```python
from build123d import *

# Parameters (mm, degrees)
SKETCH_1_W             = 372.5
SKETCH_1_H             = 50
SM_BASE_FLANGE_1_DEPTH = 8
OTHER_START            = -25
OTHER_1_DEPTH          = 50
OTHER_1_2_DEPTH        = 50
CHAMFER_1_SIZE         = 10
CUT_EXTRUDE_1_DEPTH    = 374.873307418
M8X1_251_D             = 6.8
M8X1_251_CSINK_D       = 8.5
M8X1_251_CSINK_ANGLE   = 90


# Read off the part's stored shape, not the designer's step: Изгиб1
# Sheet-metal steps are written as plain solids
with BuildPart() as part:
    # Sketch 1 → Базовая кромка1 (new body)
    with BuildSketch(Plane(origin=(0, 0, 0), x_dir=(1, 0, 0), z_dir=(0, 1, 0))):
        with Locations((-186.25, 0)):
            Rectangle(SKETCH_1_W, SKETCH_1_H)
    extrude(amount=SM_BASE_FLANGE_1_DEPTH)

    # Other 1 outline → Other 1 (cut)
    with BuildSketch(Plane.XY.offset(OTHER_START)):
        with BuildLine():
            Line((-306.372583002, 8), (-309.68629166, 4.68629166))
            ThreePointArc((-309.68629166, 4.68629166), (-314.877065168, 1.217927687), (-321, 2.25e-07))
            Line((-321, 2.25e-07), (0, 0))
            Line((0, 0), (0, 8))
            Line((0, 8), (-306.372583002, 8))
        make_face()
    extrude(amount=OTHER_1_DEPTH, mode=Mode.SUBTRACT)

    # Other 1 2 outline → Other 1 2 (add)
    with BuildSketch(Plane.XY.offset(OTHER_START)):
        with BuildLine():
            Line((-321, 8.000000225), (-306.372583002, 8))
            Line((-306.372583002, 8), (-296.715728655, 17.656854152))
            ThreePointArc((-296.715728655, 17.656854152), (-294.120341909, 19.391036132), (-291.058874503, 19.999999862))
            Line((-291.058874503, 19.999999862), (0, 20))
            Line((0, 20), (0, 28))
            Line((0, 28), (-291.058874503, 27.999999862))
            ThreePointArc((-291.058874503, 27.999999862), (-297.181809368, 26.782072393), (-302.372582904, 23.313708401))
            Line((-302.372582904, 23.313708401), (-315.343145909, 10.343145909))
            ThreePointArc((-315.343145909, 10.343145909), (-317.938532627, 8.608963948), (-321, 8.000000225))
        make_face()
    extrude(amount=OTHER_1_2_DEPTH)

    # Фаска1
    chamfer_1_edges = [part.edges().sort_by_distance(p)[0] for p in [
        (-372.5, 4, -25),
        (-372.5, 4, 25),
    ]]
    chamfer(chamfer_1_edges, length=CHAMFER_1_SIZE)

    # Эскиз4 → Вытянуть1 (cut, through all)
    with BuildSketch(Plane(origin=(0, 8, 0), x_dir=(1, 0, 0), z_dir=(0, 1, 0))):
        with BuildLine():
            Line((-348.5, 8.5), (-372.5, 8.5))
            Line((-372.5, 8.5), (-372.5, -8.5))
            Line((-372.5, -8.5), (-348.5, -8.5))
            ThreePointArc((-348.5, -8.5), (-340, 0), (-348.5, 8.5))
        make_face()
    extrude(amount=-CUT_EXTRUDE_1_DEPTH, mode=Mode.SUBTRACT)

    # Зеркальное отражение1: part across plane


with BuildPart() as part_1:
    add(part.part)
    add(part.part.mirror(Plane(origin=(0, 28, -25), x_dir=(0, 0, 1), z_dir=(-1, 0, 0))))

    # Отверстие обработанное метчиком M8x1.251 (through all)
    with Locations(Plane.XZ.offset(-20)):
        with Locations((-238.5, 17.5), (-238.5, 1.5), (-213.5, 1.5), (-213.5, 17.5), (-153, -8), (-153, 8), (-169, -8), (213.5, 1.5), (238.5, 1.5), (238.5, 17.5), (213.5, 17.5), (169, -8), (153, -8), (153, 8)):
            CounterSinkHole(M8X1_251_D / 2, M8X1_251_CSINK_D / 2, counter_sink_angle=M8X1_251_CSINK_ANGLE)


solid = part_1.part
```
For this review, take the finished solid that the model builds, in its own axes (mm). A direction names the side the tool comes from. Give positions to 0.01 mm unless a question says otherwise; leave off trailing zeros. Write each loop counter-clockwise with the first axis right and the second up, starting at its lowest first coordinate (ties: lowest second). Pieces come first, ordered by that corner, then holes.
Item 1: Insertion check: P1, Ø2, axis at y = 11.5, z = -12, coming from the -X side; P2, Ø5.5, axis at x = 153, z = -8, coming from the +Y side; P3, Ø25, axis at x = -350, z = 12, coming from the +Y side; P4, Ø1.5, axis at y = 13, z = 13.5, coming from the -X side. Each pin has a flat end and moves straight along its axis. Give the tip position at first contact, or say it passes through.
Item 2: Machinability: for faces 1 (the face through (-341, 8, -6)), 2 (the face through (341, 8, -6)), 3 (the face through (341, 0, -6)), 4 (the face through (314.8, 1.25, -0.35)), which of the approach directions +Z, -Z, +X, -X, +Y, -Y give a long, thin tool a straight path to every point of the face, cutting with its end or side? Answer none if there is none.
Item 3: Wall thickness on probe 1 along Z at (x, y) = (-153, 22.5); probe 2 along Z at (x, y) = (-213.5, 23.25); probe 3 along X at (y, z) = (23.5, -8): over which ranges is each line inside the solid? List them lowest first.
Item 4: Take a section at A-A (x = -73). Give the boundary of the cut face in (y, z).
Established:
1. P1: stops at x = -315.19
1. P2: passes through
1. P3: stops at y = 8
1. P4: stops at x = -313.44
2. face 1: +Z, -Z, -X, +Y
2. face 2: +Z, -Z, +X, +Y
2. face 3: +Z, -Z, +X, -X, -Y
2. face 4: +Z, -Z, -Y
3. probe 1: z = -25 to -11.4, -4.6 to 4.6, 11.4 to 25
3. probe 2: z = -25 to -1.9, 4.9 to 14.1, 20.9 to 25
3. probe 3: x = -302.18 to -172.4, -165.6 to -156.4, -149.6 to 149.6, 156.4 to 165.6, 172.4 to 302.18
4. outline: (20, -25) - (28, -25) - (28, 25) - (20, 25) - close
